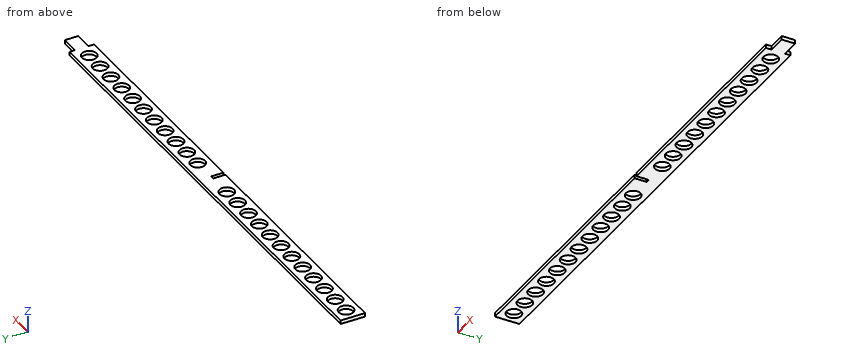
```python
from build123d import *

# Parameters (mm, degrees)
SKETCH1_W               = 415
SKETCH1_H               = 20
BOSS_EXTRUDE1_DEPTH     = 3
SKETCH2_R               = 6
SKETCH2_W               = 15
SKETCH2_H               = 4.5
SKETCH2_W_2             = 3
SKETCH2_H_2             = 10
CUT_EXTRUDE1_DEPTH      = 1
CUT_EXTRUDE1_DEPTH_BACK = 4


with BuildPart() as part:
    # Sketch1 → Boss-Extrude1 (new body)
    with BuildSketch(Plane.XY):
        with Locations((-207.5, 10)):
            Rectangle(SKETCH1_W, SKETCH1_H)
    extrude(amount=BOSS_EXTRUDE1_DEPTH)

    # Sketch2 → Cut-Extrude1 (cut, two sides)
    with BuildSketch(Plane.XY.offset(3)) as cut_extrude1_sk:
        with Locations((-405, 10)):
            Circle(SKETCH2_R)
        with Locations((-389, 10)):
            Circle(SKETCH2_R)
        with Locations((-373, 10)):
            Circle(SKETCH2_R)
        with Locations((-357, 10)):
            Circle(SKETCH2_R)
        with Locations((-341, 10)):
            Circle(SKETCH2_R)
        with Locations((-325, 10)):
            Circle(SKETCH2_R)
        with Locations((-309, 10)):
            Circle(SKETCH2_R)
        with Locations((-293, 10)):
            Circle(SKETCH2_R)
        with Locations((-277, 10)):
            Circle(SKETCH2_R)
        with Locations((-261, 10)):
            Circle(SKETCH2_R)
        with Locations((-245, 10)):
            Circle(SKETCH2_R)
        with Locations((-229, 10)):
            Circle(SKETCH2_R)
        with Locations((-26, 10)):
            Circle(SKETCH2_R)
        with Locations((-42, 10)):
            Circle(SKETCH2_R)
        with Locations((-58, 10)):
            Circle(SKETCH2_R)
        with Locations((-74, 10)):
            Circle(SKETCH2_R)
        with Locations((-90, 10)):
            Circle(SKETCH2_R)
        with Locations((-106, 10)):
            Circle(SKETCH2_R)
        with Locations((-122, 10)):
            Circle(SKETCH2_R)
        with Locations((-138, 10)):
            Circle(SKETCH2_R)
        with Locations((-154, 10)):
            Circle(SKETCH2_R)
        with Locations((-170, 10)):
            Circle(SKETCH2_R)
        with Locations((-186, 10)):
            Circle(SKETCH2_R)
        with Locations((-7.5, 17.75)):
            Rectangle(SKETCH2_W, SKETCH2_H)
        with Locations((-7.5, 2.25)):
            Rectangle(SKETCH2_W, SKETCH2_H)
        with Locations((-207.5, 5)):
            Rectangle(SKETCH2_W_2, SKETCH2_H_2)
    extrude(amount=CUT_EXTRUDE1_DEPTH, mode=Mode.SUBTRACT)
    extrude(cut_extrude1_sk.sketch, amount=-CUT_EXTRUDE1_DEPTH_BACK, mode=Mode.SUBTRACT)


solid = part.part
```
CAD build for the part. Positions are in the model's coordinates, mm. Round coordinates to 2 decimals unless told otherwise and drop trailing zeros. Order: outer loops, then holes, each group sorted by start corner. A loop starts at its lowest first (then second) coordinate and runs counter-clockwise, first axis right, second up. Notation, with made-up numbers: (51.25, -4) - (93.25, -4) arc R35 cw to (93.25, 28) - close; hole circle Ø5 at (4.5, 33.5). An arc over 180 degrees is marked (long way). Answer as CSV lines item,"result". Start each with the question number.
1. Saw through at B-B, the plane z = 1.6. Count the separate pieces of the cut face and the enclosed holes in it, and give its area (3 significant figures).
2. Saw through at A-A, the plane x = -389. Write the cut outline in (y, z).
3. Drill centre lines: L1, parallel to Y at x = -138, z = 1.35; L2, parallel to Y at x = -248, z = 1.65; L3, parallel to X at y = 18, z = 0.65. Where is each one in solid material? Low to high. Write a range as [from, to].
Model answer:
1,separate pieces,"1"
1,enclosed holes,"23"
1,area,"5,530 mm²"
2,outline,"(0, 0) - (4, 0) - (4, 3) - (0, 3) - close; (16, 0) - (20, 0) - (20, 3) - (16, 3) - close"
3,L1,"y = [0, 4], [16, 20]"
3,L2,"y = [0, 4.8], [15.2, 20]"
3,L3,"x = [-415, -15]"
